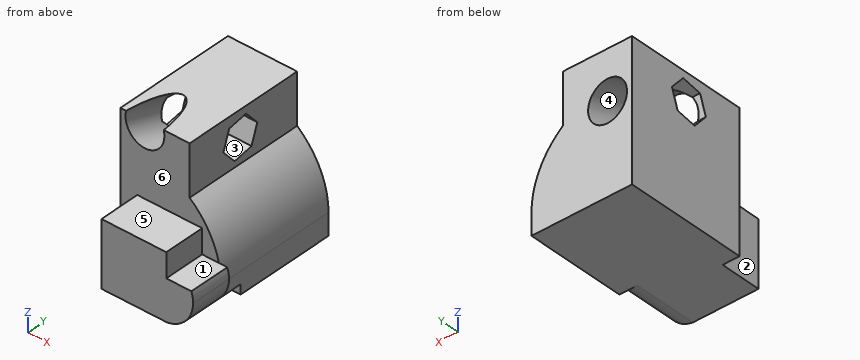
from build123d import *

# Parameters (mm, degrees)
F0_W          = 62.0737820864
F0_H          = 75.7545232773
F1_DEPTH      = 53.8003519177
F2_W          = 42.7050869912
F2_H          = 75.7545232773
F3_DEPTH      = 31.1090257019
F5_DEPTH      = 50.4763200879
F6_R          = 11.9924338382
F7_DEPTH      = 57.1455173194
F7_DEPTH_BACK = 70.5328881741
F8_W          = 23.3642431419
F8_H          = 25
F9_DEPTH      = 25.2702012658
F11_DEPTH     = 39.0601754189
F12_T1_DEPTH  = 176.500859237


# Not quite as in the source:
# - a fillet or chamfer that OpenCascade refuses, or shapes differently, is made with other operations: its cross-section is extruded or revolved along the edge and cut away or added


with BuildPart() as f1:
    # F0 (on Top) → F1 (new body)
    with BuildSketch(Plane.XY):
        with Locations((3.4712180495, 2.1439939737)):
            Rectangle(F0_W, F0_H)
    extrude(amount=F1_DEPTH)

    # F2 (on face) → F3 (join)
    with BuildSketch(Plane.XY.offset(53.8003519177)):
        with Locations((-6.2131294981, 2.1439939737)):
            Rectangle(F2_W, F2_H)
    extrude(amount=F3_DEPTH)

    # F4 (on face) → F5 (cut)
    with BuildSketch(Plane.YZ.offset(15.1394139975)):
        Polygon((7.902597892, 59.6732337929), (11.9554921985, 71.1383074522), (4.0528943065, 80.3807537101), (-7.902597892, 78.1581263088), (-11.9554921985, 66.6930526495), (-4.0528943065, 57.4506063916), align=None)
    extrude(amount=-F5_DEPTH, mode=Mode.SUBTRACT)

    # F6 (on face) → F7 (cut, two sides)
    with BuildSketch(Plane(origin=(0, -11.726481381, 4.1453017256), x_dir=(1, 0, 0), z_dir=(0, -0.9428250988, 0.3332879132))) as f7_sk:
        with Locations((-12.427136302, 65.1199892163)):
            Circle(F6_R)
    extrude(amount=-F7_DEPTH, mode=Mode.SUBTRACT)
    extrude(f7_sk.sketch, amount=F7_DEPTH_BACK, mode=Mode.SUBTRACT)

    # F8 (on face) → F9 (join)
    with BuildSketch(Plane.XZ.offset(35.7332676649)):
        with Locations((46.1902306637, 12.5)):
            Rectangle(F8_W, F8_H)
        Polygon((-17.1276477654, 40), (-17.1276477654, 0), (34.5081090927, 0), (34.5081090927, 25), (22.8723522346, 25), (22.8723522346, 40), align=None)
    extrude(amount=F9_DEPTH)

    # F10 (on face) → F11 (cut)
    with BuildSketch(Plane.XZ.offset(61.0034689307)):
        with BuildLine():
            ThreePointArc((38.360852409, 25), (39.1514020631, 21.9206371156), (39.417401399, 18.7525637448))
            ThreePointArc((39.417401399, 18.7525637448), (34.8909952827, 6.443784061), (23.4685587384, 0))
            Line((23.4685587384, 0), (57.8723522346, 0))
            Line((57.8723522346, 0), (57.8723522346, 25))
            Line((57.8723522346, 25), (38.360852409, 25))
        make_face()
    extrude(amount=-F11_DEPTH, mode=Mode.SUBTRACT)

    # F12: fillet of radius 51.606941339 on 1 edges, made by hand

    # F12_s2 → F12_t1 (cut)
    with BuildSketch(Plane.XZ.offset(-140.7675915721)):
        with BuildLine():
            ThreePointArc((34.5081090927, 13.5018175338), (29.4145726879, 35.8575674831), (15.1394139975, 53.8003519177))
            Line((15.1394139975, 53.8003519177), (34.5081090927, 53.8003519177))
            Line((34.5081090927, 53.8003519177), (34.5081090927, 13.5018175338))
        make_face()
    extrude(amount=F12_T1_DEPTH, mode=Mode.SUBTRACT)


solid = f1.part
Check sheet for the modelled part. Datum: model origin and axes. Units: mm. Face numbers are marked on the shaded views. A direction names the side the tool comes from. Round coordinates to 2 decimals unless told otherwise and drop trailing zeros. Write each loop counter-clockwise with the first axis right and the second up, starting at its lowest first coordinate (ties: lowest second). Pieces come first, ordered by that corner, then holes. Notation, with made-up numbers: (62, 73.25) -> (85, 73.25) arc R18 ccw to (85, 81.25) -> close; hole circle Ø1 at (66, 32.5). An arc over 180 degrees is marked (long way). Answer as CSV lines item,"result". Start each with the question number.
1) Release check for a two-part mould opening along Z. For the marked faces 4, 5 and 6 record: pulls with the +Z half, pulls with the -Z half, needs draft (parallel to the pull), parting line crosses it, or undercut.
2) Section check B-B on y = -38.5. Enter the section's corners in (x, z), and give its area (3 significant figures).
3) Material ranges on line 1 (Z direction, x = -7, y = -50.5); line 2 (Y direction, x = 27, z = 28); line 3 (X direction, y = -30, z = 68.5), recorded low to high. Write a range as from..to.
4) Section check A-A on x = 2. Enter the section's corners in (y, z), and give its area (3 significant figures).
5) Section check D-D on z = 61. State how many separate pieces and enclosed holes the cut face has, and give its area (3 significant figures).
6) Section check C-C on z = 15.5. Enter the section's corners in (x, y).
7) Go/stop test with flat-tipped pins: P1, Ø7.5, axis at y = -46, z = 27.5, coming from the -X side; P2, Ø5, axis at x = 38, z = 12, coming from the +Y side; P3, Ø2, axis at y = 13, z = 17.5, coming from the +X side. Record where each tip stops, or that it passes through.
8) Tool access check on the marked faces 1, 2 and 3. Record the directions out of +Z, -Z, +X, -X, +Y, -Y that give a thin tool (end or side, any length) a straight path to the whole face; none if there is none.
Found:
1,face 4,"undercut"
1,face 5,"pulls with the +Z half"
1,face 6,"needs draft"
2,outline,"(-17.13, 0) -> (23.47, 0) arc R19 ccw to (38.36, 25) -> (22.87, 25) -> (22.87, 40) -> (-17.13, 40) -> close"
2,area,"1,940 mm^2"
3,line 1,"z = 0..40"
3,line 2,"y = -35.73..40.02"
3,line 3,"x = -27.57..-18.16, -6.7..15.14"
4,outline,"(-61, 0) -> (40.02, 0) -> (40.02, 84.91) -> (-35.73, 84.91) -> (-35.73, 40) -> (-61, 40) -> close; hole (-11.96, 66.69) -> (-4.05, 57.45) -> (7.9, 59.67) -> (11.96, 71.14) -> (4.05, 80.38) -> (-7.9, 78.16) -> close"
4,area,"7,060 mm^2"
5,separate pieces,"3"
5,enclosed holes,"0"
5,area,"1,790 mm^2"
6,outline,"(-27.57, -35.73) -> (-17.13, -35.73) -> (-17.13, -61) -> (39.14, -61) -> (39.14, -35.73) -> (34.47, -35.73) -> (34.47, 40.02) -> (-27.57, 40.02) -> close"
7,P1,"stops at x = -17.13"
7,P2,"stops at y = -35.73"
7,P3,"stops at x = 34.42"
8,face 1,"+Z, +X, -Y"
8,face 2,"+Z, -Z, -X, -Y"
8,face 3,"+X, -X"
